Autodesk Inventor part; units mm, degrees
ref_plane "YZ Plane" through (0, 0, 0) normal (1, 0, 0) x (0, 1, 0)
ref_plane "XZ Plane" through (0, 0, 0) normal (0, 1, 0) x (-1, 0, 0)
ref_plane "XY Plane" through (0, 0, 0) normal (0, 0, 1) x (1, 0, 0)
sketch "Sketch1" plane through (0, 0, 0) normal (0, 1, 0) x (-1, 0, 0)
  line L0 (0, 0) -> (9.91, 0)
  line L1 (9.91, 0) -> (9.91, -19.22)
  line L2 (9.91, -19.22) -> (0, -19.22)
  line L3 (0, -19.22) -> (0, 0)
  dimension "d0" = 19.22
  dimension "d1" = 9.91
extrude "Extrusion1" add sketch "Sketch1" along normal blind 258.6
sketch "Sketch2" plane through (0, 0, 0) normal (0, -1, 0) x (1, 0, 0)
  line L0 (0, -1.7) -> (-7, -1.7)
  line L1 (-7, -1.7) -> (-7, -5.84)
  line L2 (-7, -5.84) -> (0, -5.84)
  line L3 (0, -5.84) -> (0, -1.7)
  line L4 (0, 0) -> (-9.91, 0)
  line L5 (0, -19.22) -> (0, 0)
  dimension "d31" = 1.7
  dimension "d32" = 4.14
  dimension "d33" = 7
extrude "Extrusion2" cut sketch "Sketch2" against normal through all
sketch "Sketch3" plane through (0, 0, 0) normal (0, -1, 0) x (1, 0, 0)
  line L0 (0, -7.54) -> (-7, -7.54)
  line L1 (-7, -7.54) -> (-7, -11.68)
  line L2 (-7, -11.68) -> (0, -11.68)
  line L3 (0, -11.68) -> (0, -7.54)
  line L4 (0, -5.84) -> (-7, -5.84)
  line L5 (-7, -5.84) -> (-7, -1.7)
  point P0 (0, 0)
  dimension "d39" = 1.7
  dimension "d40" = 4.14
extrude "Extrusion3" cut sketch "Sketch3" against normal through all
sketch "Sketch4" plane through (0, 0, 0) normal (0, -1, 0) x (1, 0, 0)
  line L0 (0, -13.38) -> (-7, -13.38)
  line L1 (-7, -13.38) -> (-7, -17.52)
  line L2 (-7, -17.52) -> (0, -17.52)
  line L3 (0, -17.52) -> (0, -13.38)
  line L4 (0, -11.68) -> (-7, -11.68)
  line L5 (-7, -11.68) -> (-7, -7.54)
  point P0 (0, 0)
  dimension "d43" = 1.7
  dimension "d44" = 4.14
extrude "Extrusion4" cut sketch "Sketch4" against normal through all
hole "Hole7" at (0, 3, -12.53) direction (-1, 0, 0) diameter 2.9 end through all counterbore diameter 6.5 counterbore depth 7
hole "Hole8" at (0, 143.4, -12.53) direction (-1, 0, 0) diameter 2.9 end through all counterbore diameter 6.5 counterbore depth 7
hole "Hole15" at (0, 255.6, -12.53) direction (-1, 0, 0) diameter 2.9 end through all counterbore diameter 6.5 counterbore depth 7
sketch "Sketch6" plane through (-9.91, 0, -19.22) normal (-1, 0, 0) x (0, 0, 1)
  line L0 (0, 0) -> (0, 258.6)
  line L1 (19.22, 0) -> (19.22, 258.6)
  line L2 (0, 138.6) -> (19.22, 138.6)
  line L3 (19.22, 138.6) -> (19.22, 111.2)
  line L4 (19.22, 111.2) -> (0, 111.2)
  line L5 (0, 111.2) -> (0, 138.6)
  line L6 (19.22, 0) -> (0, 0)
  dimension "d158" = 111.2
  dimension "d159" = 138.6
extrude "Extrusion6" cut sketch "Sketch6" against normal blind 1.45 contours L0 L2 L1 L4
sketch "Sketch7" plane through (-9.91, 258.6, -19.22) normal (-1, 0, 0) x (0, 0, 1)
  line L0 (0, -120) -> (0, 0)
  line L1 (19.22, -120) -> (19.22, 0)
  line L2 (0, -6.2) -> (19.22, -6.2)
  line L3 (19.22, -6.2) -> (19.22, -33.6)
  line L4 (19.22, -33.6) -> (0, -33.6)
  line L5 (0, -33.6) -> (0, -6.2)
  line L6 (19.22, -258.6) -> (0, -258.6)
  dimension "d162" = 225
  dimension "d163" = 252.4
extrude "Extrusion7" cut sketch "Sketch7" against normal blind 1.45
properties part number "6089-111_FF_right_heatsink"
Work out the finished part from the listing and answer in its coordinate system (mm). A direction names the side the tool comes from. Round coordinates to 2 decimals unless told otherwise and drop trailing zeros. Loops run counter-clockwise (first coordinate to the right, second up) from the corner with the lowest first, then second, coordinate; pieces in that order, holes last. Notation, with made-up numbers: (11, 0.5) -> (52, 0.5) arc R12 cw to (52, 16.5) -> close; hole circle Ø1 at (-17, 31). An arc over 180 degrees is marked (long way). Use one line per item in the form item = value.
(1) A tool of negligible diameter and unlimited length cuts with its end or side. For faces 1 (the flat face through (-6, 258.6, -7)), 2 (the flat face through (-8.46, 239, -10)), 3 (the flat face through (-3, 72, -13.38)), from which of +Z, -Z, +X, -X, +Y, -Y can it reach the whole face along a straight path? Write none if from no direction.
Answer list:
face_1 = +Z, -Z, +X, -X, +Y
face_2 = +Z, -Z, -X
face_3 = +X, +Y, -Y
(2) For a pull along Z with two mould halves and no side action, classify faces 4 (the flat face through (-5, 127, 0)), 5 (the flat face through (-3, 199, -13.38)), 6 (the flat face through (-4, 127, -5.84)), 7 (the flat face through (-9.91, 255, -9)) as released by +Z, released by -Z, zero draft, split by the parting line, or undercut.
Answer list:
face_4 = released by +Z
face_5 = undercut
face_6 = undercut
face_7 = zero draft
(3) Flat-ended cylindrical pins translate along their axes: P1, Ø0.7, axis at x = -9, z = -13.5, coming from the -Y side; P2, Ø2, axis at y = 124.5, z = -7.5, coming from the -X side; P3, Ø3, axis at x = -3, z = -14.5, coming from the +Y side; P4, Ø3, axis at y = 218.5, z = -10, coming from the +X side. Find the tip coordinate at first contact, or state that the pin passes through.
Answer list:
P1 = 0
P2 = -8.46
P3 = 252.46
P4 = -7
(4) Find section B-B on y = 149. Give the vertices of the cut face in (x, z).
Answer list:
outline = (-9.91, -19.22) -> (0, -19.22) -> (0, -17.52) -> (-7, -17.52) -> (-7, -13.38) -> (0, -13.38) -> (0, -11.68) -> (-7, -11.68) -> (-7, -7.54) -> (0, -7.54) -> (0, -5.84) -> (-7, -5.84) -> (-7, -1.7) -> (0, -1.7) -> (0, 0) -> (-9.91, 0) -> close
(5) Find section A-A on x = -3.5. Give the vertices of the cut face in (y, z), then the cut area to 3 significant figures.
Answer list:
outline = (0, -19.22) -> (258.6, -19.22) -> (258.6, -17.52) -> (0, -17.52) -> close; (0, -7.54) -> (258.6, -7.54) -> (258.6, -5.84) -> (0, -5.84) -> close; (0, -1.7) -> (258.6, -1.7) -> (258.6, 0) -> (0, 0) -> close; (6.14, -13.38) -> (140.26, -13.38) arc R3.25 cw to (140.26, -11.68) -> (6.14, -11.68) arc R3.25 cw to start; (146.54, -13.38) -> (252.46, -13.38) arc R3.25 cw to (252.46, -11.68) -> (146.54, -11.68) arc R3.25 cw to start
area = 1,730 mm2
(6) Straight lines are drawn through the part: line 1 (Y direction, x = -7.9, z = -12.53); line 2 (Y direction, x = -9.1, z = -12.53); line 3 (Z direction, x = -1.75, y = 212). For each, find the intervals that lie inside material, in ascending order.
Answer list:
line_1 = 0 to 1.55, 4.45 to 141.95, 144.85 to 254.15, 257.05 to 258.6
line_2 = 0 to 1.55, 4.45 to 111.2, 138.6 to 141.95, 144.85 to 225, 252.4 to 254.15, 257.05 to 258.6
line_3 = -19.22 to -17.52, -13.38 to -11.68, -7.54 to -5.84, -1.7 to 0
